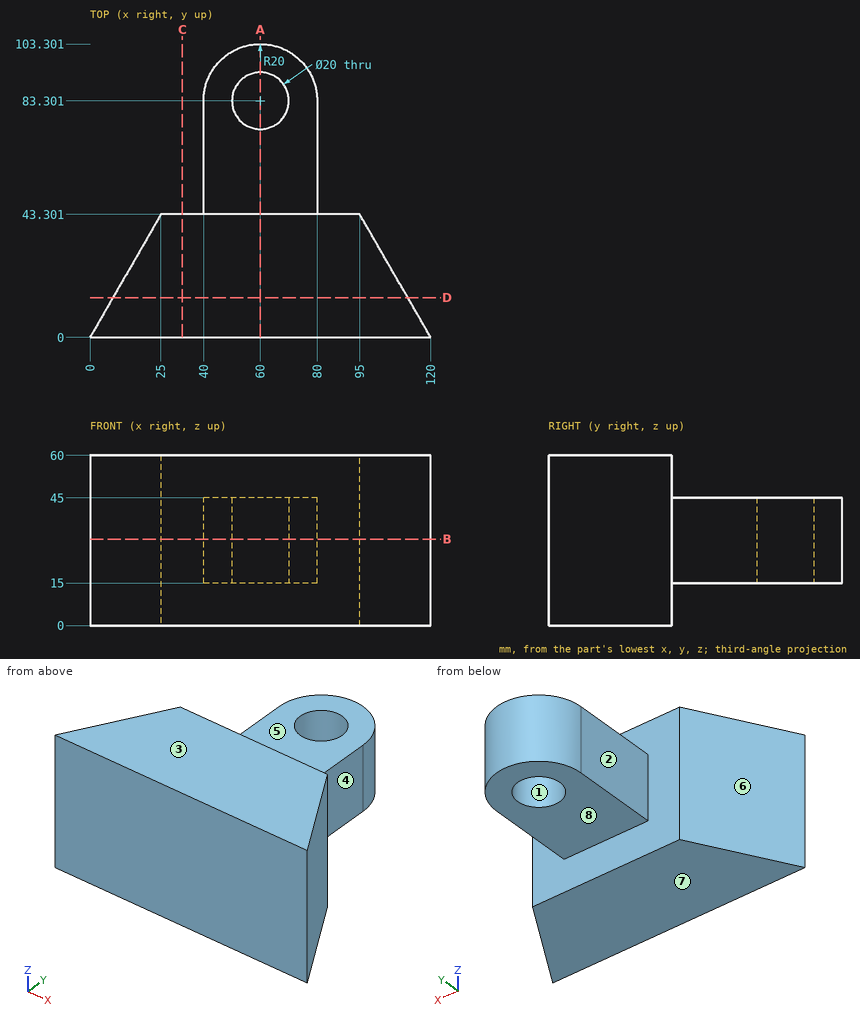
Study the drawing (mm; zero at the part's minimum x, y, z) and answer. A direction names the side the tool comes from. Coordinates: 2 decimals unless noted, no trailing zeros. Loops run counter-clockwise (first coordinate to the right, second up) from the corner with the lowest first, then second, coordinate; pieces in that order, holes last. Notation, with made-up numbers: M 66.5,50.25 L 96.5,50.25 A32 cw 96.5,83.25 Z; hole C 82.5,21 d7. An arc over 180 degrees is marked long. Answer in a Markdown table with one row per item. Add a question column.
1. Consider L1, parallel to Y at x = 60, z = 29.25; L2, parallel to X at y = 44.5, z = 43; L3, parallel to Y at x = 43, z = 56. Determine where each line is inside the solid, lowest interval first.
2. Find section A-A, the plane x = 60. Write down the section's boundary in (y, z), then the cut area to 3 significant figures.
3. The mould has two halves that part along X. Classify the marked faces 1, 2 and 3: pulls with the +X half, pulls with the -X half, needs draft (parallel to the pull), parting line crosses it, or undercut.
4. Flat-ended cylindrical pins translate along their axes: P1, Ø4, axis at y = 72, z = 22, coming from the +X side; P2, Ø24, axis at y = 54, z = 31, coming from the -X side; P3, Ø5, axis at y = 29, z = 21.5, coming from the -X side; P4, Ø8, axis at y = 91, z = 51, coming from the +X side. Find the tip coordinate at first contact, or state that the pin passes through.
5. Find section C-C, the plane x = 32.5. Write down the section's boundary in (y, z).
6. Find section D-D, the plane y = 14. Write down the section's boundary in (x, z).
7. Find section B-B, the plane z = 30.5. Write down the section's boundary in (x, y), then the cut area to 3 significant figures.
8. A tool of negligible diameter and unlimited length cuts with its end or side. For the marked faces 4, 5, 6, 7 and 8, from which of +Z, -Z, +X, -X, +Y, -Y can it reach the whole face along a straight path? Write none if from no direction.
Reported:
| question | item | result |
|---|---|---|
| 1 | L1 | y = 0 to 73.3, 93.3 to 103.3 |
| 1 | L2 | x = 40 to 80 |
| 1 | L3 | y = 0 to 43.3 |
| 2 | outline | M 0,0 L 43.3,0 L 43.3,15 L 73.3,15 L 73.3,45 L 43.3,45 L 43.3,60 L 0,60 Z; M 93.3,15 L 103.3,15 L 103.3,45 L 93.3,45 Z |
| 2 | area | 3,800 mm^2 |
| 3 | face 1 | undercut |
| 3 | face 2 | pulls with the -X half |
| 3 | face 3 | needs draft |
| 4 | P1 | stops at x = 80 |
| 4 | P2 | stops at x = 24.25 |
| 4 | P3 | stops at x = 15.3 |
| 4 | P4 | passes through |
| 5 | outline | M 0,0 L 43.3,0 L 43.3,60 L 0,60 Z |
| 6 | outline | M 8.08,0 L 111.92,0 L 111.92,60 L 8.08,60 Z |
| 7 | outline | M 0,0 L 120,0 L 95,43.3 L 80,43.3 L 80,83.3 A20 ccw 40,83.3 L 40,43.3 L 25,43.3 Z; hole C 60,83.3 d20 |
| 7 | area | 6,030 mm^2 |
| 8 | face 4 | +Z, -Z, +X, +Y |
| 8 | face 5 | +Z, +X, -X, +Y |
| 8 | face 6 | +Z, -Z, -X, +Y |
| 8 | face 7 | -Z, +X, -X, +Y, -Y |
| 8 | face 8 | -Z, +X, -X, +Y |
